Autodesk Inventor part; units mm, degrees
ref_plane "YZ Plane" through (0, 0, 0) normal (1, 0, 0) x (0, 1, 0)
ref_plane "XZ Plane" through (0, 0, 0) normal (0, 1, 0) x (-1, 0, 0)
ref_plane "XY Plane" through (0, 0, 0) normal (0, 0, 1) x (1, 0, 0)
sketch "Boceto1" plane through (0, 0, 0) normal (0, 1, 0) x (-1, 0, 0)
  line L0 (-2.95, -6.65) -> (2.95, -6.65)
  line L1 (2.95, -6.65) -> (2.95, 6.65)
  line L2 (2.95, 6.65) -> (-2.95, 6.65)
  line L3 (-2.95, 6.65) -> (-2.95, -6.65)
  line L4 (-2.95, -6.65) -> (2.95, 6.65) construction
  line L5 (2.95, -6.65) -> (-2.95, 6.65) construction
  line L6 (4.45, 8.15) -> (4.45, -8.15)
  line L7 (4.45, -8.15) -> (-4.45, -8.15)
  line L8 (-4.45, -8.15) -> (-4.45, 8.15)
  line L9 (-4.45, 8.15) -> (4.45, 8.15)
  point P0 (0, 0)
  dimension "d0" = 5.9
  dimension "d1" = 13.3
  dimension "d2" = 1.5
extrude "Extrusión1" add sketch "Boceto1" along normal blind 8.7
sketch "Boceto2" plane through (0, 8.7, 0) normal (0, 1, 0) x (1, 0, 0)
  line L0 (4.45, -8.15) -> (4.45, 8.15)
  line L1 (4.45, 8.15) -> (-4.45, 8.15)
  line L2 (-4.45, 8.15) -> (-4.45, -8.15)
  line L3 (-4.45, -8.15) -> (4.45, -8.15)
  line L4 (2.95, 6.65) -> (2.95, -6.65)
  line L5 (2.95, -6.65) -> (-2.95, -6.65)
  line L6 (-2.95, -6.65) -> (-2.95, 6.65)
  line L7 (-2.95, 6.65) -> (2.95, 6.65)
  line L8 (-5.95, -9.65) -> (-5.95, 9.65)
  line L9 (-5.95, 9.65) -> (5.95, 9.65)
  line L10 (5.95, 9.65) -> (5.95, -9.65)
  line L11 (5.95, -9.65) -> (-5.95, -9.65)
  point P0 (0, 0)
  dimension "d5" = 1.5
extrude "Extrusión2" add sketch "Boceto2" against normal blind 1 contours L8 L9 L10 L11
fillet "Empalme1" radius 2 4 edges at (5.95, 8.2, 9.65) (-5.95, 8.2, 9.65) (5.95, 8.2, -9.65) (-5.95, 8.2, -9.65)
fillet "Empalme2" radius 1 4 edges at (4.45, 3.85, 8.15) (-4.45, 3.85, 8.15) (4.45, 3.85, -8.15) (-4.45, 3.85, -8.15)
sketch "Boceto3" plane through (0, 0, 0) normal (0, -1, 0) x (1, 0, 0)
  line L0 (0, 0) -> (0, -1.25)
  line L1 (0, -1.25) -> (4.45, -1.25)
  line L2 (4.45, 7.15) -> (4.45, -7.15)
  line L3 (0, 0) -> (0, 1.25)
  line L4 (0, 1.25) -> (4.45, 1.25)
  dimension "d10" = 1.25
  dimension "d11" = 1.25
extrude "Extrusión3" cut sketch "Boceto3" against normal blind 3.5
split "Dividir1" plane through (0, 0, 0) removes the side toward (0, 0, -1)
properties part number "PIeza Conector USB"
Here's how the part is built. I have some questions about the finished solid (model axes, mm). A direction names the side the tool comes from. Round coordinates to 2 decimals unless told otherwise and drop trailing zeros. Order: outer loops, then holes, each group sorted by start corner. A loop starts at its lowest first (then second) coordinate and runs counter-clockwise, first axis right, second up. Notation, with made-up numbers: (18, 16) -> (25, 16) arc R22 ccw to (25, 24) -> close; hole circle Ø7 at (-40, 75.5). An arc over 180 degrees is marked (long way). Return JSON: item names as keys, results as strings.
Q1. If we section it at A-A on y = 6.75: List the corners of the cut face in (x, z) for me, plus the area to 3 significant figures.
Filled sheet:
{"outline": "(-4.45, 0) -> (-2.95, 0) -> (-2.95, 6.65) -> (2.95, 6.65) -> (2.95, 0) -> (4.45, 0) -> (4.45, 7.15) arc R1 ccw to (3.45, 8.15) -> (-3.45, 8.15) arc R1 ccw to (-4.45, 7.15) -> close", "area": "32.9 mm^2"}
Q2. For pin 1 Ø4 at (y, z) = (2, 3) entering from +X; pin 2 Ø3 at (x, y) = (-0.5, 6) entering from -Z; pin 3 Ø1 at (y, z) = (4, 2.5) entering from -X, each with a flat end and sliding along its axis, tell me the tip position at first contact or that it passes through.
Filled sheet:
{"pin 1": "stops at x = 4.45", "pin 2": "stops at z = 6.65", "pin 3": "stops at x = -4.45"}
Q3. If we section it at C-C on x = 3.25: List the corners of the cut face in (y, z) for me.
Filled sheet:
{"outline": "(0, 1.25) -> (3.5, 1.25) -> (3.5, 0) -> (8.7, 0) -> (8.7, 9.65) -> (7.7, 9.65) -> (7.7, 8.15) -> (0, 8.15) -> close"}
Q4. If we section it at D-D on z = 7.5: List the corners of the cut face in (x, y) for me.
Filled sheet:
{"outline": "(-5.95, 7.7) -> (-4.39, 7.7) -> (-4.39, 0) -> (4.39, 0) -> (4.39, 7.7) -> (5.95, 7.7) -> (5.95, 8.7) -> (-5.95, 8.7) -> close"}
Q5. If we mould it in two halves opening along X, with no side actions, what happens to faces 1 (the flat face through (-2.95, 4, 3)), 2 (the flat face through (0, 4, 8.15)), 3 (the cylindrical face through (-4.165, 3.904, 7.849)), 4 (the flat face through (2.95, 4, 3))? For each: released by +X, released by -X, zero draft, split by the parting line, or undercut.
Filled sheet:
{"face 1": "undercut", "face 2": "zero draft", "face 3": "released by -X", "face 4": "undercut"}
Q6. I need wall thicknesses on line 1 along X through (y, z) = (1.5, 5.75); line 2 along Y through (x, z) = (-4.5, 1.5); line 3 along X through (y, z) = (5, 7). Which ranges of each line are inside material? Lowest first, please. Write a range as from..to.
Filled sheet:
{"line 1": "x = -4.45..-2.95, 2.95..4.45", "line 2": "y = 7.7..8.7", "line 3": "x = -4.45..4.45"}
Q7. Which directions (+Z, -Z, +X, -X, +Y, -Y) give clear straight access to the entire face, cutting with the end or side of a thin tool? Please do faces 5 (the flat face through (0, 4, 6.65)), 6 (the flat face through (-4.45, 4, 4)), 7 (the flat face through (0, 7.7, 9)), 8 (the flat face through (4, 2, 1.25)).
Filled sheet:
{"face 5": "-Z, +Y, -Y", "face 6": "+Z, -Z, -X, -Y", "face 7": "+Z, -Y", "face 8": "-Z, +X, -Y"}
Q8. If we section it at B-B on z = 2: List the corners of the cut face in (x, y) for me, plus the area to 3 significant figures.
Filled sheet:
{"outline": "(-5.95, 7.7) -> (-4.45, 7.7) -> (-4.45, 0) -> (-2.95, 0) -> (-2.95, 8.7) -> (-5.95, 8.7) -> close; (2.95, 0) -> (4.45, 0) -> (4.45, 7.7) -> (5.95, 7.7) -> (5.95, 8.7) -> (2.95, 8.7) -> close", "area": "29.1 mm^2"}
